Here's how the part is built. I have some questions about the finished solid (model axes, mm). A direction names the side the tool comes from. Give positions to 0.01 mm unless a question says otherwise; leave off trailing zeros. Order: outer loops, then holes, each group sorted by start corner. A loop starts at its lowest first (then second) coordinate and runs counter-clockwise, first axis right, second up. Notation, with made-up numbers: M 62,-26 L 73,-26 A14 ccw 73,-20 Z; hole C 78.25,0 d10. An arc over 180 degrees is marked long. Use one line per item in the form item = value.
from build123d import *

# Parameters (mm, degrees)
SKETCH1_W                = 1.96
SKETCH1_H                = 300
BOSS_EXTRUDE1_DEPTH      = 152
BOSS_EXTRUDE1_DEPTH_BACK = 152
SKETCH3_R                = 76.2
SKETCH3_R_2              = 75.2


with BuildPart() as part:
    # Sketch1 → Revolve1 (revolve)
    with BuildSketch(Plane.XY, mode=Mode.PRIVATE) as revolve1_sk:
        with Locations((77.18, 150)):
            Rectangle(SKETCH1_W, SKETCH1_H)
    revolve(revolve1_sk.sketch.rotate(Axis((0, 204.615384615, 0), (0, -1, 0)), 90), axis=Axis((0, 204.615384615, 0), (0, -1, 0)))

    # Sketch3 → Boss-Extrude1 (add, two sides: drawn at the far end of the back side and taken through both)
    with BuildSketch(Plane(origin=(0, 300, 0), x_dir=(1, 0, 0), z_dir=(0, 1, 0)).offset(-BOSS_EXTRUDE1_DEPTH_BACK)):
        with Locations(Location((0, 0, 0), (0, 0, 270))):
            Circle(SKETCH3_R)
        with Locations(Location((0, 0, 0), (0, 0, 270))):
            Circle(SKETCH3_R_2, mode=Mode.SUBTRACT)
    extrude(amount=BOSS_EXTRUDE1_DEPTH + BOSS_EXTRUDE1_DEPTH_BACK)


solid = part.part
Q1. I'm going to push flat-ended pins straight in: pin 1 Ø1.5 at (x, y) = (-58.5, 116.5) entering from +Z; pin 2 Ø5 at (x, y) = (60, 176.5) entering from -Z; pin 3 Ø6 at (y, z) = (89, -22.5) entering from +X. Where does each tip first touch, or does it pass through?
Found:
pin_1 = 52.67
pin_2 = -52.94
pin_3 = 75.69
Q2. Thinking about a two-plate mould opening in X: for faces 1 (the face through (76.301, 152.1, -16.944)), 2 (the face through (74.388, 75.036, -16.519)), 3 (the face through (-50.4, 452, 56.1)), which applies, +X half, -X half, draft (parallel to the pull), parting line (faces both ways), or undercut?
Found:
face_1 = parting line
face_2 = undercut
face_3 = draft
Q3. I want a section at A-A on x = 0. Write out the boundary of the cut face in (y, z).
Found:
outline = M 0,-78.16 L 300,-78.16 L 300,-76.2 L 452,-76.2 L 452,-75.2 L 148,-75.2 L 148,-76.2 L 0,-76.2 Z; M 0,76.2 L 148,76.2 L 148,75.2 L 452,75.2 L 452,76.2 L 300,76.2 L 300,78.16 L 0,78.16 Z
Q4. I want a section at B-B on z = 0. Write out the boundary of the cut face in (x, y).
Found:
outline = M -78.16,0 L -76.2,0 L -76.2,148 L -75.2,148 L -75.2,452 L -76.2,452 L -76.2,300 L -78.16,300 Z; M 75.2,148 L 76.2,148 L 76.2,0 L 78.16,0 L 78.16,300 L 76.2,300 L 76.2,452 L 75.2,452 Z
Q5. I want a section at C-C on y = 320.5. Write out the boundary of the cut face in (x, z).
Found:
outline = C 0,0 d152.4; hole C 0,0 d150.4
Q6. I want a section at D-D on y = 231. Write out the boundary of the cut face in (x, z), then the cut area to 3 significant figures.
Found:
outline = C 0,0 d156.32; hole C 0,0 d150.4
area = 1,430 mm²
Q7. I need wall thicknesses on L1, parallel to X at y = 331, z = 0; L2, parallel to Z at x = 3, y = 222.5; L3, parallel to X at y = 37, z = 0. Which ranges of each line are inside material? Lowest first, please.
Found:
L1 = -76.2 to -75.2, 75.2 to 76.2
L2 = -78.1 to -75.14, 75.14 to 78.1
L3 = -78.16 to -76.2, 76.2 to 78.16
Q8. On a 3-axis mill with a long thin cutter (end or side, diameter ignored), from which of +Z, -Z, +X, -X, +Y, -Y can I reach the whole of each face in a straight line? I mean faces 4 (the face through (22.588, 297.872, 71.727)), 5 (the face through (17, 300, -75)), 6 (the face through (-50.4, 148, 56.1)). Say none if no direction works.
Found:
face_4 = +Y, -Y
face_5 = +Y
face_6 = -Y
